Autodesk Fusion 360 part; units mm, degrees
sketch "Sketch1" plane through (0, 0, 0) normal (0, 0, 1) x (1, 0, 0)
  line L0 (13.335, 13.335) -> (-13.335, 13.335)
  line L1 (-13.335, 13.335) -> (-13.335, -13.335)
  line L2 (-13.335, -13.335) -> (13.335, -13.335)
  line L3 (13.335, -13.335) -> (13.335, 13.335)
  line L4 (13.335, 13.335) -> (-13.335, -13.335) construction
  line L5 (-13.335, 13.335) -> (13.335, -13.335) construction
  line L6 (16.51, 16.51) -> (-16.51, 16.51)
  line L7 (-16.51, 16.51) -> (-16.51, -16.51)
  line L8 (-16.51, -16.51) -> (16.51, -16.51)
  line L9 (16.51, -16.51) -> (16.51, 16.51)
  line L10 (16.51, 16.51) -> (-16.51, -16.51) construction
  line L11 (-16.51, 16.51) -> (16.51, -16.51) construction
  dimension "d1" = 26.67
  dimension "d2" = 26.67
  dimension "d3" = 33.02
  dimension "d4" = 33.02
extrude "Extrude1" add sketch "Sketch1" along normal blind 25.4
sketch "Sketch2" plane through (0, 0, 0) normal (0, 0, 1) x (1, 0, 0)
  line L0 (25.4, 25.4) -> (-25.4, 25.4)
  line L1 (-25.4, 25.4) -> (-25.4, -25.4)
  line L2 (-25.4, -25.4) -> (25.4, -25.4)
  line L3 (25.4, -25.4) -> (25.4, 25.4)
  line L4 (25.4, 25.4) -> (-25.4, -25.4) construction
  line L5 (-25.4, 25.4) -> (25.4, -25.4) construction
  dimension "d7" = 50.8
  dimension "d8" = 50.8
extrude "Extrude2" add sketch "Sketch2" against normal blind 2.54
fillet "Fillet1" radius 2.54 4 edges at (16.51, 0, 0) (0, -16.51, 0) (-16.51, 0, 0) (0, 16.51, 0)
sketch "Sketch4" plane through (0, 0, 0) normal (0, 0, 1) x (-1, 0, 0)
  line L0 (-25.4, 25.4) -> (-25.4, -25.4)
  line L1 (-25.4, -25.4) -> (25.4, -25.4)
  line L2 (25.4, -25.4) -> (25.4, 25.4)
  line L3 (25.4, 25.4) -> (-25.4, 25.4)
  line L4 (-19.05, -19.05) -> (-19.05, 19.05)
  line L5 (-19.05, 19.05) -> (19.05, 19.05)
  line L6 (19.05, 19.05) -> (19.05, -19.05)
  line L7 (19.05, -19.05) -> (-19.05, -19.05)
  circle A0 centre (20.828, -20.828) radius 1.778
  circle A1 centre (-20.828, -20.828) radius 1.778
  circle A2 centre (20.828, 20.828) radius 1.778
  circle A3 centre (-20.828, 20.828) radius 1.778
  dimension "d14" = 3.556
  dimension "d15" = 3.556
  dimension "d16" = 3.556
  dimension "d17" = 3.556
  dimension "d18" = 4.572
  dimension "d19" = 4.572
  dimension "d20" = 4.572
  dimension "d21" = 4.572
  dimension "d22" = 4.572
  dimension "d23" = 4.572
  dimension "d25" = 4.572
  dimension "d41" = 4.572
extrude "Extrude3" cut sketch "Sketch4" against normal blind 2.54 contours A0 | A1 | A2 | A3
sketch "Sketch5" plane through (-16.51, 0, 0) normal (-1, 0, 0) x (0, -1, 0)
  line L0 (-16.51, 2.54) -> (16.51, 2.54)
  line L1 (16.51, 2.54) -> (16.51, 25.4)
  line L2 (16.51, 25.4) -> (-16.51, 25.4)
  line L3 (-16.51, 25.4) -> (-16.51, 2.54)
  circle A0 centre (0.6022, 12.7) radius 1.778
  dimension "d28" = 3.556
  dimension "d29" = 12.7
  dimension "d30" = 15.9078
extrude "Extrude4" cut sketch "Sketch5" against normal blind 5.08 contours A0
sketch "Sketch7" plane through (16.51, 0, 0) normal (1, 0, 0) x (0, 1, 0)
  line L0 (-16.51, 2.54) -> (16.51, 2.54)
  line L1 (16.51, 2.54) -> (16.51, 25.4)
  line L2 (16.51, 25.4) -> (-16.51, 25.4)
  line L3 (-16.51, 25.4) -> (-16.51, 2.54)
  circle A0 centre (-0.0337, 12.7) radius 1.778
  dimension "d37" = 3.556
  dimension "d38" = 12.7
extrude "Extrude6" cut sketch "Sketch7" against normal blind 5.08 contours A0
Design review of the part built by this model. Coordinates are the model's own, in mm. A direction names the side the tool comes from. Coordinates: 2 decimals unless noted, no trailing zeros. Write each loop counter-clockwise with the first axis right and the second up, starting at its lowest first coordinate (ties: lowest second). Pieces come first, ordered by that corner, then holes. Notation, with made-up numbers: (76, 1) - (124, 1) arc R23 cw to (124, 11) - close; hole circle Ø7 at (28, 25). An arc over 180 degrees is marked (long way). Use one line per item in the form item = value.
Q1. The part is to be moulded in two halves that separate along X. For faces 5 (the flat face through (-13.335, 0, 15)), 6 (the flat face through (25.4, 0, -1)), 7 (the flat face through (-25.4, 0, -1)), say which applies: +X half, -X half, draft (parallel to the pull), parting line (faces both ways), or undercut.
Taken from the geometry:
face_5 = undercut
face_6 = +X half
face_7 = -X half
Q2. For probe 1 along X at (y, z) = (1, 15.75) (3 decimals); probe 2 along Z at (x, y) = (0.5, -4.5), list the stretches that pass through material, from the lowest coordinate up.
Taken from the geometry:
probe_1 = -16.51 to -13.335, 13.335 to 16.51
probe_2 = -2.54 to 0
Q3. Consider section D-D (x = -20). Write out the cut boundary in (y, z), plus the area to 3 significant figures.
Taken from the geometry:
outline = (-25.4, -2.54) - (-22.4, -2.54) - (-22.4, 0) - (-25.4, 0) - close; (-19.25, -2.54) - (19.25, -2.54) - (19.25, 0) - (-19.25, 0) - close; (22.4, -2.54) - (25.4, -2.54) - (25.4, 0) - (22.4, 0) - close
area = 113 mm^2
Q4. Consider section C-C (z = 20.75). Write out the cut boundary in (x, y) (3 decimals).
Taken from the geometry:
outline = (-16.51, -16.51) - (16.51, -16.51) - (16.51, 16.51) - (-16.51, 16.51) - close; hole (-13.335, -13.335) - (13.335, -13.335) - (13.335, 13.335) - (-13.335, 13.335) - close
Q5. Insertion check: pin 1 Ø4 at (x, z) = (-8, 4.5) entering from -Y; pin 2 Ø1.5 at (x, y) = (-10, 11) entering from +Z; pin 3 Ø1 at (x, z) = (-6, 2.5) entering from +Y. Each pin has a flat end and moves straight along its axis. Give the tip position at first contact, or say it passes through.
Taken from the geometry:
pin_1 = -16.51
pin_2 = 0
pin_3 = 16.57
Q6. Consider section B-B (y = 14). Write out the cut boundary in (x, z), plus the area to 3 significant figures.
Taken from the geometry:
outline = (-25.4, -2.54) - (25.4, -2.54) - (25.4, 0) - (19.05, 0) arc R2.54 cw to (16.51, 2.54) - (16.51, 25.4) - (-16.51, 25.4) - (-16.51, 2.54) arc R2.54 cw to (-19.05, 0) - (-25.4, 0) - close
area = 971 mm^2
Q7. Machinability: for faces 1 (the flat face through (0, 16.51, 14)), 2 (the flat face through (16.51, 0, 16)), 3 (the flat face through (0, -16.51, 14)), 4 (the flat face through (22, 0, 0)), which of the approach directions +Z, -Z, +X, -X, +Y, -Y give a long, thin tool a straight path to every point of the face, cutting with its end or side? Answer none if there is none.
Taken from the geometry:
face_1 = +Z, +X, -X, +Y
face_2 = +Z, +X, +Y, -Y
face_3 = +Z, +X, -X, -Y
face_4 = +Z
Q8. Consider section A-A (z = 12.7). Write out the cut boundary in (x, y) (3 decimals).
Taken from the geometry:
outline = (-16.51, -16.51) - (16.51, -16.51) - (16.51, -1.812) - (13.335, -1.812) - (13.335, -13.335) - (-13.335, -13.335) - (-13.335, -2.38) - (-16.51, -2.38) - close; (-16.51, 1.176) - (-13.335, 1.176) - (-13.335, 13.335) - (13.335, 13.335) - (13.335, 1.744) - (16.51, 1.744) - (16.51, 16.51) - (-16.51, 16.51) - close
